The listing builds one solid part. Answer for the finished solid, in the listing's coordinates (mm). A direction names the side the tool comes from. Round coordinates to 2 decimals unless told otherwise and drop trailing zeros. Write each loop counter-clockwise with the first axis right and the second up, starting at its lowest first coordinate (ties: lowest second). Pieces come first, ordered by that corner, then holes. Notation, with made-up numbers: (-30, 19.25) - (12, 19.25) arc R24 cw to (12, 38.25) - close; hole circle Ø1 at (27.5, 19.25). An arc over 180 degrees is marked (long way). Use a Markdown table: item, result. Add a question column.
1) Find the intervals of material crossed by probe 1 along Z at (x, y) = (-66.5, 8.75); probe 2 along X at (y, z) = (6, -162.5) (3 decimals); probe 3 along Z at (x, y) = (-19.5, 5.5), in increasing order. Write a range as from..to.
2) A tool of negligible diameter and unlimited length cuts with its end or side. For faces 1 (the flat face through (-83, 6, -400.05)), 2 (the flat face through (-6, 6, -412.75)), 3 (the flat face through (-67, 6, -683.006)), from which of +Z, -Z, +X, -X, +Y, -Y can it reach the whole face along a straight path? Write none if from no direction.
3) Each of these flat-tipped pins is pushed along its axis until it touches: P1, Ø2, axis at x = -49.5, y = 11, coming from the -Z side; P2, Ø2, axis at y = 10.5, z = -394.5, coming from the +X side. Where does it stop, or does it pass through?
4) A cutting plane is placed at B-B (y = 5.5). State how many separate pieces and enclosed holes the cut face has, then the cut area to 3 significant figures.
5) A cutting plane is placed at A-A (z = -168.5). Give the vertices of the cut face in (x, y) (3 decimals).
6) Determine the mould class of faces 4 (the flat face through (-79.375, 6, -749)), 5 (the flat face through (-67, 6, -695.706)), 6 (the flat face through (-54, 0, -374)) for opening direction X: +X half, -X half, draft (parallel to the pull), parting line (faces both ways), or undercut.
Autodesk Inventor part; units mm, degrees
ref_plane "YZ Plane" through (0, 0, 0) normal (1, 0, 0) x (0, 1, 0)
ref_plane "XZ Plane" through (0, 0, 0) normal (0, 1, 0) x (-1, 0, 0)
ref_plane "XY Plane" through (0, 0, 0) normal (0, 0, 1) x (1, 0, 0)
sketch "Sketch1" plane through (0, 0, 0) normal (0, 1, 0) x (-1, 0, 0)
  line L0 (0, 0) -> (88.9, 0)
  line L1 (88.9, -762) -> (0, -762)
  line L2 (0, -762) -> (0, 0)
  line L3 (88.9, 0) -> (0, 0) construction
  line L4 (0, 0) -> (0, -50.8) construction
  line L5 (88.9, 0) -> (88.9, -762)
  dimension "d0" = 88.9
  dimension "d3" = 50.8
  dimension "d47" = 762
extrude "Extrusion3" add sketch "Sketch1" along normal blind 12.7
sketch "Sketch2" plane through (0, 12.7, 0) normal (0, 1, 0) x (1, 0, 0)
  line L0 (0, 762) -> (-88.9, 762) construction
  line L1 (-44.45, 762) -> (666.75, 762) construction
  line L2 (-41.275, 63.5) -> (-47.625, 63.5)
  line L3 (-47.625, 63.5) -> (-47.625, 673.1)
  line L4 (-47.625, 673.1) -> (-41.275, 673.1)
  line L5 (-41.275, 673.1) -> (-41.275, 63.5)
  line L6 (-44.45, 63.5) -> (-44.45, 0) construction
  line L7 (-88.9, 0) -> (0, 0) construction
  dimension "d21" = 6.35
  dimension "d22" = 609.6
  dimension "d25" = 63.5
extrude "Extrusion4" cut sketch "Sketch2" against normal through all
sketch "Sketch3" plane through (0, 0, 0) normal (0, -1, 0) x (1, 0, 0)
  line L0 (-41.275, -673.1) -> (-41.275, -63.5) construction
  line L1 (-41.275, -63.5) -> (-22.225, -63.5) construction
  line L2 (-47.625, -63.5) -> (-41.275, -63.5) construction
  line L3 (-44.45, -63.5) -> (-44.45, 0) construction
  line L4 (-47.625, -63.5) -> (-66.675, -63.5) construction
  line L5 (-28.575, -57.15) -> (-15.875, -57.15)
  line L6 (-15.875, -57.15) -> (-15.875, -69.85)
  line L7 (-15.875, -69.85) -> (-28.575, -69.85)
  line L8 (-28.575, -69.85) -> (-28.575, -57.15)
  line L9 (-28.575, -57.15) -> (-15.875, -69.85) construction
  line L10 (-15.875, -57.15) -> (-28.575, -69.85) construction
  line L11 (-60.325, -57.15) -> (-73.025, -57.15)
  line L12 (-73.025, -57.15) -> (-73.025, -69.85)
  line L13 (-73.025, -69.85) -> (-60.325, -69.85)
  line L14 (-60.325, -69.85) -> (-60.325, -57.15)
  line L15 (-60.325, -57.15) -> (-73.025, -69.85) construction
  line L16 (-73.025, -57.15) -> (-60.325, -69.85) construction
  line L17 (-28.575, -660.4) -> (-15.875, -660.4)
  line L18 (-15.875, -660.4) -> (-15.875, -673.1)
  line L19 (-15.875, -673.1) -> (-28.575, -673.1)
  line L20 (-28.575, -673.1) -> (-28.575, -660.4)
  line L21 (-28.575, -660.4) -> (-15.875, -673.1) construction
  line L22 (-15.875, -660.4) -> (-28.575, -673.1) construction
  line L23 (-60.325, -660.4) -> (-73.025, -660.4)
  line L24 (-73.025, -660.4) -> (-73.025, -673.1)
  line L25 (-73.025, -673.1) -> (-60.325, -673.1)
  line L26 (-60.325, -673.1) -> (-60.325, -660.4)
  line L27 (-60.325, -660.4) -> (-73.025, -673.1) construction
  line L28 (-73.025, -660.4) -> (-60.325, -673.1) construction
  line L29 (-47.625, -673.1) -> (-41.275, -673.1) construction
  line L30 (-28.575, -673.1) -> (-60.325, -673.1) construction
  line L31 (-44.45, -673.1) -> (-44.45, -695.706) construction
  line L32 (-44.45, -673.1) -> (-21.844, -673.1) construction
  line L33 (-28.575, -695.706) -> (-28.575, -683.006)
  line L34 (-15.875, -695.706) -> (-28.575, -695.706)
  line L35 (-15.875, -683.006) -> (-15.875, -695.706)
  line L36 (-15.875, -683.006) -> (-28.575, -695.706) construction
  line L37 (-28.575, -683.006) -> (-15.875, -683.006)
  line L38 (-28.575, -683.006) -> (-15.875, -695.706) construction
  line L39 (-60.325, -695.706) -> (-60.325, -683.006)
  line L40 (-60.325, -683.006) -> (-73.025, -683.006)
  line L41 (-73.025, -683.006) -> (-73.025, -695.706)
  line L42 (-60.325, -683.006) -> (-73.025, -695.706) construction
  line L43 (-73.025, -683.006) -> (-60.325, -695.706) construction
  line L44 (-73.025, -695.706) -> (-60.325, -695.706)
  line L45 (-28.575, -695.706) -> (-60.325, -695.706) construction
  line L46 (0, -762) -> (-88.9, -762) construction
  line L47 (-44.45, -762) -> (-44.45, -755.65) construction
  line L48 (-44.45, -755.65) -> (-15.875, -755.65) construction
  line L49 (-15.875, -755.65) -> (-9.525, -755.65)
  line L50 (-9.525, -755.65) -> (-9.525, -742.95)
  line L51 (-9.525, -742.95) -> (-15.875, -742.95)
  line L52 (-15.875, -742.95) -> (-15.875, -755.65)
  line L53 (-73.025, -755.65) -> (-79.375, -755.65)
  line L54 (-79.375, -755.65) -> (-79.375, -742.95)
  line L55 (-79.375, -742.95) -> (-73.025, -742.95)
  line L56 (-73.025, -742.95) -> (-73.025, -755.65)
  point P0 (0, 0)
  point P1 (-22.225, -666.75)
  point P2 (-66.675, -666.75)
  point P3 (-22.225, -689.356)
  point P4 (-66.675, -689.356)
  point P5 (-21.844, -695.706)
  dimension "d26" = 19.05
  dimension "d27" = 12.7
  dimension "d28" = 12.7
  dimension "d29" = 12.7
  dimension "d30" = 12.7
  dimension "d33" = 12.7
  dimension "d34" = 12.7
  dimension "d35" = 12.7
  dimension "d36" = 12.7
  dimension "d37" = 22.606
  dimension "d38" = 90
  dimension "d39" = 12.7
  dimension "d40" = 12.7
  dimension "d41" = 12.7
  dimension "d42" = 12.7
  dimension "d43" = 6.35
  dimension "d44" = 28.575
  dimension "d45" = 6.35
  dimension "d46" = 12.7
extrude "Extrusion5" cut sketch "Sketch3" against normal through all
sketch "Sketch4" plane through (0, 0, 0) normal (0, -1, 0) x (1, 0, 0)
  line L0 (-88.9, -406.4) -> (0, -406.4) construction
  line L1 (-88.9, -400.05) -> (-76.2, -400.05)
  line L2 (-76.2, -400.05) -> (-76.2, -412.75)
  line L3 (-76.2, -412.75) -> (-88.9, -412.75)
  line L4 (-88.9, -400.05) -> (-88.9, -412.75)
  line L5 (0, -400.05) -> (-12.7, -400.05)
  line L6 (-12.7, -400.05) -> (-12.7, -412.75)
  line L7 (-12.7, -412.75) -> (0, -412.75)
  line L8 (0, -400.05) -> (0, -412.75)
  line L9 (-15.875, -742.95) -> (-15.875, -755.65) construction
  line L10 (-79.375, -755.65) -> (-73.025, -755.65) construction
  line L11 (-15.875, -755.65) -> (-73.025, -755.65) construction
  line L12 (-28.575, -69.85) -> (-28.575, -57.15) construction
  line L13 (-28.575, -57.15) -> (-60.325, -57.15) construction
  line L14 (-44.45, -57.15) -> (-44.45, -755.65) construction
  point P0 (-44.45, -406.4)
  dimension "d49" = 12.7
  dimension "d52" = 12.7
extrude "Extrusion6" cut sketch "Sketch4" against normal through all
fillet "Fillet1" radius 3.175 6 edges at (0, 12.7, -200.025) (-44.45, 12.7, 0) (-88.9, 12.7, -200.025) (0, 12.7, -587.375) (-44.45, 12.7, -762) (-88.9, 12.7, -587.375)
fillet "Fillet2" radius 3.175 1 edges at (-44.45, 0, -762)
sketch "Sketch5" plane through (0, 12.7, 0) normal (0, 1, 0) x (1, 0, 0)
  line L0 (-85.725, 3.175) -> (-85.725, 400.05) construction
  line L1 (-3.175, 400.05) -> (-3.175, 3.175) construction
  line L2 (-85.725, 57.15) -> (-3.175, 57.15) construction
  line L3 (-3.175, 57.15) -> (-3.175, 3.175) construction
  line L4 (-3.175, 3.175) -> (-85.725, 3.175) construction
  line L5 (-85.725, 3.175) -> (-85.725, 57.15) construction
  line L6 (-85.725, 57.15) -> (-4.458, 3.175) construction
  line L7 (-70.4915, 17.4625) -> (-19.6915, 17.4625) construction
  line L8 (-19.6915, 17.4625) -> (-19.6915, 42.8625) construction
  line L9 (-19.6915, 42.8625) -> (-70.4915, 42.8625) construction
  line L10 (-70.4915, 42.8625) -> (-70.4915, 17.4625) construction
  line L11 (-70.4915, 17.4625) -> (-19.6915, 42.8625) construction
  line L12 (-19.6915, 17.4625) -> (-70.4915, 42.8625) construction
  circle A0 centre (-70.4915, 42.8625) radius 3
  circle A1 centre (-19.6915, 42.8625) radius 3
  circle A2 centre (-19.6915, 17.4625) radius 3
  circle A3 centre (-70.4915, 17.4625) radius 3
  point P0 (0, 0)
  point P1 (-45.0915, 30.1625)
  dimension "d64" = 50.8
  dimension "d65" = 25.4
  dimension "d66" = 6
  dimension "d67" = 6
  dimension "d68" = 6
  dimension "d69" = 6
extrude "Extrusion7" cut sketch "Sketch5" against normal through all
properties part number "Arm Base" material "PVC-Piping"
Entries:
| question | item | result |
|---|---|---|
| 1 | probe 1 | z = -762..-695.71, -683.01..-673.1, -660.4..-69.85, -57.15..0 |
| 1 | probe 2 | x = -88.9..-47.625, -41.275..0 |
| 1 | probe 3 | z = -762..-695.71, -683.01..-673.1, -660.4..-69.85, -57.15..-45.86, -39.87..-20.46, -14.47..0 |
| 2 | face 1 | -X, +Y, -Y |
| 2 | face 2 | +X, +Y, -Y |
| 2 | face 3 | +Y, -Y |
| 3 | P1 | stops at z = -761.96 |
| 3 | P2 | stops at x = 0 |
| 4 | separate pieces | 1 |
| 4 | enclosed holes | 13 |
| 4 | area | 62,300 mm² |
| 5 | outline | (-88.9, 0) - (-47.625, 0) - (-47.625, 12.7) - (-85.725, 12.7) arc R3.175 ccw to (-88.9, 9.525) - close; (-41.275, 0) - (0, 0) - (0, 9.525) arc R3.175 ccw to (-3.175, 12.7) - (-41.275, 12.7) - close |
| 6 | face 4 | undercut |
| 6 | face 5 | undercut |
| 6 | face 6 | draft |
